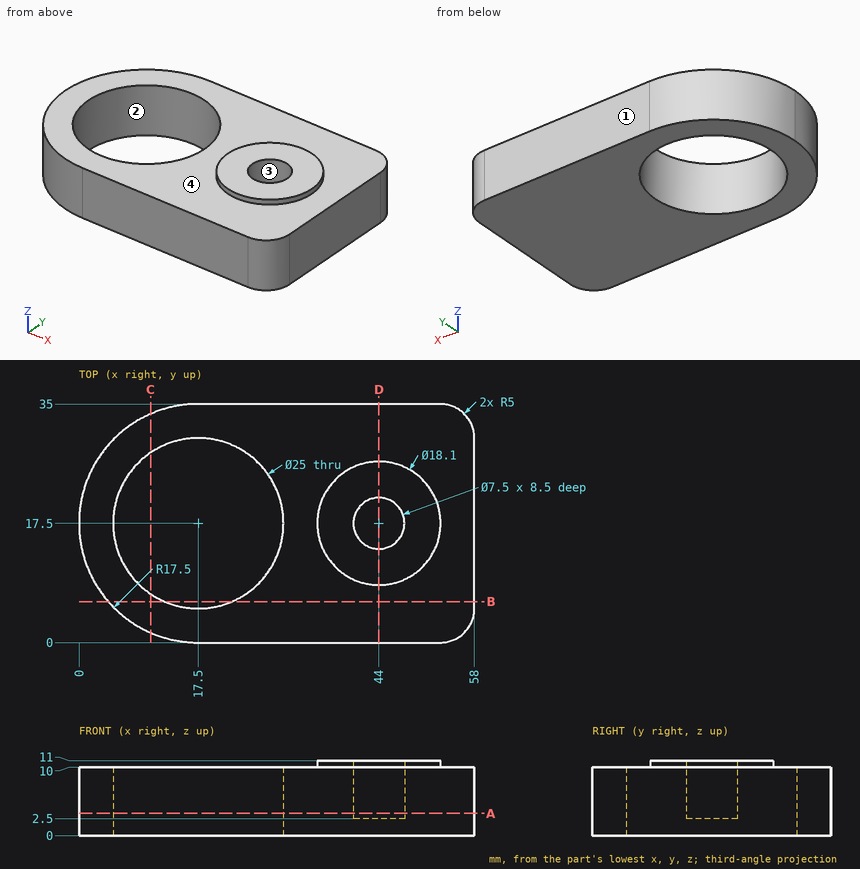
The figure shows three views and two pictorial views of one solid part (mm, origin at its lowest corner). Answer the questions. Coordinates: 2 decimals unless noted, no trailing zeros. Loops run counter-clockwise (first coordinate to the right, second up) from the corner with the lowest first, then second, coordinate; pieces in that order, holes last. Notation, with made-up numbers: M 13.5,-1.75 L 71.5,-1.75 A17 ccw 71.5,24.25 Z; hole C 65.5,-1.5 d4. An arc over 180 degrees is marked long. Answer as CSV lines item,"result". Start each with the question number.
(1) The part is cut by section B-B (y = 6). Give the vertices of the cut face in (x, z), and give its area (3 significant figures).
(2) The part is cut by section D-D (x = 44). Give the vertices of the cut face in (y, z).
(3) Find the intervals of material crossed by L1, parallel to Z at x = 33, y = 10; L2, parallel to Y at x = 43.5, z = 9.25; L3, parallel to X at y = 8, z = 1.5, in increasing order. Write a range as [from, to].
(4) The part is cut by section C-C (x = 10.5). Give the vertices of the cut face in (y, z).
(5) The part is cut by section A-A (z = 3.25). Give the vertices of the cut face in (x, y).
(6) The mould has two halves that part along Y. Classify the marked faces 1, 2, 3 and 4: pulls with the +Y half, pulls with the -Y half, needs draft (parallel to the pull), parting line crosses it, or undercut.
(7) Given pin 1 (3 mm diameter, centred on x = 8.5, z = 2.5, fed in from +Y); pin 2 (1 mm diameter, centred on x = 30, y = 11, fed in from +Z); pin 3 (4 mm diameter, centred on y = 26.5, z = 2, fed in from -X); pin 4 (20 mm diameter, centred on x = 17.5, y = 17.5, fed in from +Z), each flat-ended and moving along its own axis, determine where each tip first touches the part or whether it passes through.
Determined:
1,outline,"M 4.31,0 L 12.6,0 L 12.6,10 L 4.31,10 Z; M 22.4,0 L 58,0 L 58,10 L 22.4,10 Z"
1,area,"439 mm2"
2,outline,"M 0,0 L 35,0 L 35,10 L 26.55,10 L 26.55,11 L 21.25,11 L 21.25,2.5 L 13.75,2.5 L 13.75,11 L 8.45,11 L 8.45,10 L 0,10 Z"
3,L1,"[0, 10]"
3,L2,"[0, 13.78], [21.22, 35]"
3,L3,"[2.8, 9.38], [25.62, 58]"
4,outline,"M 1.46,0 L 7.14,0 L 7.14,10 L 1.46,10 Z; M 27.86,0 L 33.54,0 L 33.54,10 L 27.86,10 Z"
5,outline,"M 0,17.5 A17.5 ccw 17.5,0 L 53,0 A5 ccw 58,5 L 58,30 A5 ccw 53,35 L 17.5,35 A17.5 ccw Z; hole C 17.5,17.5 d25; hole C 44,17.5 d7.5"
6,face 1,"pulls with the +Y half"
6,face 2,"undercut"
6,face 3,"undercut"
6,face 4,"needs draft"
7,pin 1,"y = 33.31"
7,pin 2,"z = 10"
7,pin 3,"x = 1.46"
7,pin 4,"through"
